Model file for the job. Use its own axes, mm. A direction names the side the tool comes from. Coordinates: 2 decimals unless noted, no trailing zeros. Order: outer loops, then holes, each group sorted by start corner. A loop starts at its lowest first (then second) coordinate and runs counter-clockwise, first axis right, second up.
from build123d import *

# Parameters (mm, degrees)
SKETCH_W        = 99.825
SKETCH_H        = 84
PAD_DEPTH       = 9
POCKET_DEPTH    = 7.5
POCKET001_DEPTH = 9
SKETCH003_R     = 1.6
POCKET002_DEPTH = 20
SKETCH006_W     = 15
SKETCH006_H     = 45
POCKET003_DEPTH = 5


with BuildPart() as pocket001:
    # Sketch → Pad (new body)
    with BuildSketch(Plane.XZ):
        Rectangle(SKETCH_W, SKETCH_H)
    extrude(amount=PAD_DEPTH)

    # Sketch001 → Pocket (cut)
    with BuildSketch(Plane.XZ.offset(9)):
        with BuildLine():
            Line((-48.4125, -33), (-48.4125, 42))
            Line((-48.4125, 42), (48.412084, 42))
            ThreePointArc((-48.4125, -33), (12.824744, -12.056942), (48.412084, 42))
        make_face()
    extrude(amount=-POCKET_DEPTH, mode=Mode.SUBTRACT)

    # Sketch002 → Pocket001 (cut)
    with BuildSketch(Plane.XZ.offset(9)):
        Polygon((-4.162717, -33), (49.9125, -33), (49.9125, 21.075217), align=None)
    extrude(amount=-POCKET001_DEPTH, mode=Mode.SUBTRACT)


with BuildPart() as pocket003:
    # Part__Mirroring: instance of Pocket001
    add(pocket001.part.mirror(Plane(origin=(0, 0, 0), x_dir=(1, 0, 0), z_dir=(0, 1, 0))))


with BuildPart() as pocket003_1:
    # Part__Mirroring placement: moved
    add(pocket003.part.moved(Location((0, -18, 0))))

    # Fusion: union Pocket001
    add(pocket001.part)

    # Sketch003 → Pocket002 (cut)
    with BuildSketch(Plane.XZ.offset(18)):
        with Locations((-35, -37.5)):
            Circle(SKETCH003_R)
        with Locations((35, -37.5)):
            Circle(SKETCH003_R)
    extrude(amount=-POCKET002_DEPTH, mode=Mode.SUBTRACT)

    # Sketch006 → Pocket003 (cut)
    with BuildSketch(Plane(origin=(-49.9125, 0, 0), x_dir=(0, -1, 0), z_dir=(-1, 0, 0))):
        with Locations((9, 19.5)):
            Rectangle(SKETCH006_W, SKETCH006_H)
    extrude(amount=-POCKET003_DEPTH, mode=Mode.SUBTRACT)


solid = pocket003_1.part
Q1. Probe line 1 (Y direction, x = -30, z = 15); line 2 (Z direction, x = 35, y = -8.25); line 3 (X direction, y = -13.25, z = -37). List the from-to ranges inside material, lowest first.
Established:
line 1: y = -18 to -16.5, -1.5 to 0
line 2: z = -42 to -39.1, -35.9 to -33, 6.16 to 11.84
line 3: x = -49.91 to -36.52, -33.48 to 33.48, 36.52 to 49.91
Q2. Cut at C-C, the plane z = -24. List the corners of the cut face in (x, y), plus the area to 3 significant figures.
Established:
outline: (-49.91, -18) - (4.84, -18) - (4.84, 0) - (-49.91, 0) - close; hole (-48.41, -16.5) - (-6.95, -16.5) - (-6.95, -1.5) - (-48.41, -1.5) - close
area: 364 mm2
Q3. Cut at D-D, the plane x = 35. List the corners of the cut face in (y, z).
Established:
outline: (-18, -42) - (0, -42) - (0, -39.1) - (-18, -39.1) - close; (-18, -35.9) - (0, -35.9) - (0, -33) - (-18, -33) - close; (-18, 6.16) - (0, 6.16) - (0, 42) - (-1.5, 42) - (-1.5, 11.84) - (-16.5, 11.84) - (-16.5, 42) - (-18, 42) - close
Q4. Drop flat-ended pins along their axis: P1, Ø2, axis at y = -5.5, z = 20, coming from the -X side; P2, Ø2.5, axis at x = -35, z = -37.5, coming from the -Y side; P3, Ø6, axis at x = 10.5, y = -9.5, coming from the +Z side; P4, Ø2, axis at y = -4.5, z = -11, coming from the +X side. Give the stop position or say it passes through.
Established:
P1: stops at x = 39.31
P2: passes through
P3: stops at z = -11.53
P4: stops at x = 18.84
Q5. Cut at B-B, the plane x = 9. List the corners of the cut face in (y, z), plus the area to 3 significant figures.
Established:
outline: (-18, -42) - (0, -42) - (0, -33) - (-18, -33) - close; (-18, -19.84) - (0, -19.84) - (0, 42) - (-1.5, 42) - (-1.5, -14.88) - (-16.5, -14.88) - (-16.5, 42) - (-18, 42) - close
area: 422 mm2
Q6. Mould opens along X. For faces 1 (the face through (33.73, -9.13, -38.47)), 2 (the face through (12.09, -9.1, -12.62)), 3 (the face through (22, -9, -33)), 4 (the face through (-49.912, -9, -19)) say: pulls with the +X half, pulls with the -X half, needs draft (parallel to the pull), parting line crosses it, or undercut.
Established:
face 1: undercut
face 2: undercut
face 3: needs draft
face 4: pulls with the -X half
Q7. Cut at A-A, the plane y = -5.5. List the corners of the cut face in (x, z).
Established:
outline: (-49.91, -42) - (49.91, -42) - (49.91, -33) - (-4.16, -33) - (49.91, 21.08) - (49.91, 42) - (48.41, 42) arc R100 cw to (-48.41, -33) - (-48.41, -3) - (-49.91, -3) - close; hole circle Ø3.2 at (-35, -37.5); hole circle Ø3.2 at (35, -37.5)
Q8. Which spindle directions (+Z, -Z, +X, -X, +Y, -Y) get a long thin tool onto all of the face, cutting with end or side? Do faces 5 (the face through (23.253, -9.126, -5.584)), 6 (the face through (-12, -16.5, 12)), 7 (the face through (0, -1, 42)). Say none if no direction does.
Established:
face 5: +X, +Y, -Y
face 6: +Z
face 7: +Z, +X, -X, +Y, -Y
